```python
from build123d import *

# Parameters (mm, degrees)
BOSS_EXTRUDE1_DEPTH = 1219.2
FILLET1_R           = 0.4064
SKETCH4_W           = 1838.4
SKETCH4_H           = 103.278519729
CUT_EXTRUDE1_DEPTH  = 60
SKETCH5_W           = 2.838427027
SKETCH5_H           = 1.970979722
CUT_EXTRUDE2_DEPTH  = 700


with BuildPart() as part:
    # Sketch3 → Boss-Extrude1 (new, symmetric)
    with BuildSketch(Plane.XY):
        Polygon((3.175, 25.4), (0, 25.4), (0, 0), (25.4, 0), (25.4, 3.175), (3.175, 3.175), align=None)
    extrude(amount=BOSS_EXTRUDE1_DEPTH, both=True)

    # Fillet1
    fillet1_edges = [part.edges().sort_by_distance(p)[0] for p in [
        (3.175, 3.175, 0),
    ]]
    fillet(fillet1_edges, radius=FILLET1_R)

    # Sketch4 → Cut-Extrude1 (cut)
    with BuildSketch(Plane.ZY):
        with Locations((-300, -26.239259864)):
            Rectangle(SKETCH4_W, SKETCH4_H)
    extrude(amount=-CUT_EXTRUDE1_DEPTH, mode=Mode.SUBTRACT)

    # Sketch5 → Cut-Extrude2 (cut)
    with BuildSketch(Plane(origin=(0, 0, 619.2), x_dir=(-1, 0, 0), z_dir=(0, 0, -1))):
        with Locations((-4.594213514, 4.160489861)):
            Rectangle(SKETCH5_W, SKETCH5_H)
    extrude(amount=-CUT_EXTRUDE2_DEPTH, mode=Mode.SUBTRACT)


solid = part.part
```
The model under review builds one solid part; all positions refer to its coordinate system, in mm. A direction names the side the tool comes from. Give positions to 0.01 mm unless a question says otherwise; leave off trailing zeros. Write each loop counter-clockwise with the first axis right and the second up, starting at its lowest first coordinate (ties: lowest second). Pieces come first, ordered by that corner, then holes. Notation, with made-up numbers: (-8.75, 37.25) - (12.25, 37.25) arc R12 cw to (12.25, 53.25) - close; hole circle Ø8 at (74.25, -6). An arc over 180 degrees is marked (long way). Answer in a Markdown table with one row per item. Add a question column.
1. We need section A-A on z = 1119. Write out the cut boundary in (x, y) (3 decimals).
2. We need section B-B on y = 12.25. Write out the cut boundary in (x, z) (3 decimals), then the cut area to 4 significant figures.
3. Draft analysis for pull direction Z (two halves, no side actions). For faces 1 (the flat face through (0, 13, 923)), 2 (the flat face through (7, 2, 1219.2)), 3 (the flat face through (7, 2, 619.2)), state which applies: +Z half, -Z half, draft (parallel to the pull), parting line (faces both ways), or undercut.
4. Tool access review of faces 4 (the flat face through (14, 3.175, 915)), 5 (the flat face through (13, 0, 923)): name each direction out of +Z, -Z, +X, -X, +Y, -Y from which nothing blocks a thin tool from reaching the whole face with its end or side.
5. Wall thickness on line 1 along X through (y, z) = (5.5, 889.5) (3 decimals): over which ranges is the line inside the solid? List them lowest first. Write a range as [from, to].
6. Insertion check: P1, Ø10, axis at x = 8.5, y = 16, coming from the -Z side; P2, Ø10, axis at x = 13.5, z = 1093.5, coming from the +Y side (3 decimals); P3, Ø3, axis at y = 5.5, z = 887, coming from the +X side (3 decimals). Each pin has a flat end and moves straight along its axis. Give the tip position at first contact, or say it passes through.
Ans:
| question | item | result |
|---|---|---|
| 1 | outline | (0, 0) - (25.4, 0) - (25.4, 3.175) - (3.175, 3.175) - (3.175, 25.4) - (0, 25.4) - close |
| 2 | outline | (0, 619.2) - (3.175, 619.2) - (3.175, 1219.2) - (0, 1219.2) - close |
| 2 | area | 1,905 mm^2 |
| 3 | face 1 | draft |
| 3 | face 2 | +Z half |
| 3 | face 3 | -Z half |
| 4 | face 4 | +Z, -Z, +X, +Y |
| 4 | face 5 | +Z, -Z, +X, -X, -Y |
| 5 | line 1 | x = [0, 3.175] |
| 6 | P1 | passes through |
| 6 | P2 | stops at y = 3.175 |
| 6 | P3 | stops at x = 3.175 |
